Verification items for the finished model (mm, model axes). Face numbers are marked on the shaded views. A direction names the side the tool comes from. Round coordinates to 2 decimals unless told otherwise and drop trailing zeros. Write each loop counter-clockwise with the first axis right and the second up, starting at its lowest first coordinate (ties: lowest second). Pieces come first, ordered by that corner, then holes. Notation, with made-up numbers: (81, 19) - (114, 19) arc R20 cw to (114, 37) - close; hole circle Ø9 at (-16, -25.5). An arc over 180 degrees is marked (long way). Answer as a JSON object with one key per item and string values.
```python
from build123d import *

# Parameters (mm, degrees)
F0_R     = 15
F0_R_2   = 25
F1_DEPTH = 25
F2_SIZE  = 5


with BuildPart() as f1:
    # F0 (on Top) → F1 (new body)
    with BuildSketch(Plane.XY):
        with BuildLine():
            Line((-23.352277, 62.976109), (-47.352277, 50.976109))
            Line((-47.352277, 50.976109), (-47.352277, -7.023891))
            Line((-47.352277, -7.023891), (-47.352277, -37.023891))
            Line((-47.352277, -37.023891), (-17.352277, -37.023891))
            Line((-17.352277, -37.023891), (-7.352277, -37.023891))
            Line((-7.352277, -37.023891), (-7.352277, -57.023891))
            Line((-7.352277, -57.023891), (119.360484, -57.023891))
            Line((119.360484, -57.023891), (119.360484, -37.023891))
            Line((119.360484, -37.023891), (159.360484, -37.023891))
            Line((159.360484, -37.023891), (159.360484, 37.976109))
            ThreePointArc((159.360484, 37.976109), (152.038154, 55.653779), (134.360484, 62.976109))
            Line((134.360484, 62.976109), (-23.352277, 62.976109))
        make_face()
        with Locations((-17.352277, -7.023891)):
            Circle(F0_R, mode=Mode.SUBTRACT)
        with Locations((47.647723, 32.976109)):
            Circle(F0_R_2, mode=Mode.SUBTRACT)
    extrude(amount=F1_DEPTH)

    # F2
    f2_edges = [f1.edges().sort_by_distance(p)[0] for p in [
        (-7.352277, -57.023891, 12.5),
        (119.360484, -57.023891, 12.5),
    ]]
    chamfer(f2_edges, length=F2_SIZE)


solid = f1.part
```
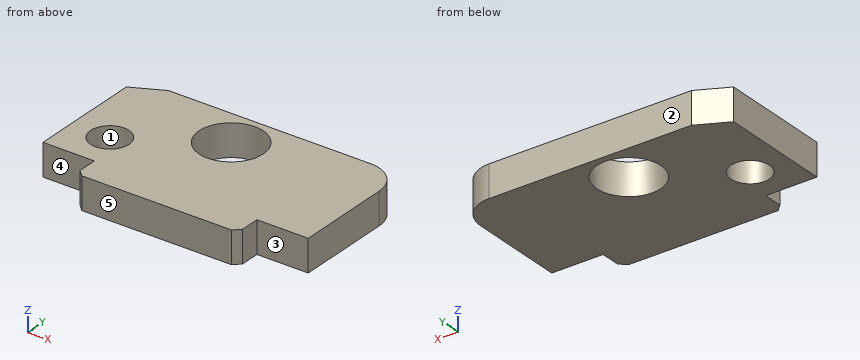
Q1. Section check C-C, the plane z = 23. Record the cut outline in (x, y), then the cut area to 3 significant figures.
Geometry check:
{"outline": "(-47.35, -37.02) - (-7.35, -37.02) - (-7.35, -52.02) - (-2.35, -57.02) - (114.36, -57.02) - (119.36, -52.02) - (119.36, -37.02) - (159.36, -37.02) - (159.36, 37.98) arc R25 ccw to (134.36, 62.98) - (-23.35, 62.98) - (-47.35, 50.98) - close; hole circle Ø30 at (-17.35, -7.02); hole circle Ø50 at (47.65, 32.98)", "area": "20,200 mm2"}
Q2. Material ranges on line 1 along X through (y, z) = (-8, 4); line 2 along X through (y, z) = (5, 6.5); line 3 along Y through (x, z) = (130.5, 11), recorded low to high. Write a range as [from, to].
Geometry check:
{"line 1": "x = [-47.35, -32.32], [-2.38, 159.36]", "line 2": "x = [-47.35, -26.32], [-8.38, 159.36]", "line 3": "y = [-37.02, 62.98]"}
Q3. Section check B-B, the plane x = 46.5. Record the cut outline in (y, z).
Geometry check:
{"outline": "(-57.02, 0) - (8, 0) - (8, 25) - (-57.02, 25) - close; (57.95, 0) - (62.98, 0) - (62.98, 25) - (57.95, 25) - close"}
Q4. Release check for a two-part mould opening along Y. For the marked faces 1, 2 and 3 record: released by +Y, released by -Y, zero draft, split by the parting line, or undercut.
Geometry check:
{"face 1": "undercut", "face 2": "released by +Y", "face 3": "released by -Y"}
Q5. Set-up check for the marked faces 4 and 5: record each of +Z, -Z, +X, -X, +Y, -Y from which the full face is reachable in a straight line by a thin tool's end or side.
Geometry check:
{"face 4": "+Z, -Z, -X, -Y", "face 5": "+Z, -Z, +X, -X, -Y"}
Q6. Section check A-A, the plane y = 4.5. Record the cut outline in (x, z).
Geometry check:
{"outline": "(-47.35, 0) - (-26.95, 0) - (-26.95, 25) - (-47.35, 25) - close; (-7.75, 0) - (159.36, 0) - (159.36, 25) - (-7.75, 25) - close"}
Q7. Gauge pin test, flat ends, axial feed: P1, Ø7.5, axis at x = -30, z = 13.5, coming from the -Y side; P2, Ø12, axis at y = -44, z = 16, coming from the +X side. Record the tip position at first contact, or that the pin passes through.
Geometry check:
{"P1": "stops at y = -37.02", "P2": "stops at x = 119.36"}
Q8. Section check D-D, the plane y = -45.5. Record the cut outline in (x, z), then the cut area to 3 significant figures.
Geometry check:
{"outline": "(-7.35, 0) - (119.36, 0) - (119.36, 25) - (-7.35, 25) - close", "area": "3,170 mm2"}
